Autodesk Inventor part; units mm, degrees
ref_plane "YZ Plane" through (0, 0, 0) normal (1, 0, 0) x (0, 1, 0)
ref_plane "XZ Plane" through (0, 0, 0) normal (0, 1, 0) x (-1, 0, 0)
ref_plane "XY Plane" through (0, 0, 0) normal (0, 0, 1) x (1, 0, 0)
sketch "Sketch1" plane through (0, 0, 0) normal (0, 0, 1) x (1, 0, 0)
  circle A0 centre (0, 0) radius 10
  arc A1 (13.8638, 0.9) -> (9.8638, 1.6449) centre (9.1431, -13.3378) ccw
  arc A2 (9.8638, -1.6449) -> (13.8638, -0.9) centre (9.1431, 13.3378) ccw
  arc A3 (13.8638, -0.9) -> (13.8638, 0.9) centre (-6.1159, 0) ccw
  line L0 (0, 0) -> (21.7354, 0) construction
  arc A4 (9.8638, -1.6449) -> (9.8638, 1.6449) centre (0, 0) ccw
  arc A5 (11.8575, 7.2397) -> (7.9696, 6.0404) centre (14.2942, -7.561) ccw
  arc A6 (12.694, 5.6459) -> (11.8575, 7.2397) centre (-5.4154, -2.8422) ccw
  arc A7 (9.4984, 3.1275) -> (12.694, 5.6459) centre (1.8975, 16.0591) ccw
  circle A8 centre (0, 0) radius 10
  arc A9 (9.4984, 3.1275) -> (7.9696, 6.0404) centre (0, 0) ccw
  arc A10 (7.1348, 11.9209) -> (4.2496, 9.0521) centre (16.1707, -0.0521) ccw
  arc A11 (8.6162, 10.8984) -> (7.1348, 11.9209) centre (-3.4743, -5.0333) ccw
  arc A12 (6.957, 7.1834) -> (8.6162, 10.8984) centre (-5.7829, 15.1014) ccw
  circle A13 centre (0, 0) radius 10
  arc A14 (6.957, 7.1834) -> (4.2496, 9.0521) centre (0, 0) ccw
  arc A15 (0.7777, 13.8712) -> (-0.4439, 9.9901) centre (14.3427, 7.4688) ccw
  arc A16 (2.5645, 13.6542) -> (0.7777, 13.8712) centre (-0.7372, -6.0714) ccw
  arc A17 (2.8218, 9.5936) -> (2.5645, 13.6542) centre (-12.1385, 10.6842) ccw
  circle A18 centre (0, 0) radius 10
  arc A19 (2.8218, 9.5936) -> (-0.4439, 9.9901) centre (0, 0) ccw
  arc A20 (-5.7577, 12.6437) -> (-5.0357, 8.6395) centre (9.2289, 13.2786) ccw
  arc A21 (-4.0747, 13.282) -> (-5.7577, 12.6437) centre (2.1687, -5.7185) ccw
  arc A22 (-1.9598, 9.8061) -> (-4.0747, 13.282) centre (-15.7133, 3.8193) ccw
  circle A23 centre (0, 0) radius 10
  arc A24 (-1.9598, 9.8061) -> (-5.0357, 8.6395) centre (0, 0) ccw
  arc A25 (-10.974, 8.5197) -> (-8.4739, 5.3097) centre (2.0009, 16.0465) ccw
  arc A26 (-9.7804, 9.8671) -> (-10.974, 8.5197) centre (4.5779, -4.0556) ccw
  arc A27 (-6.2924, 7.7721) -> (-9.7804, 9.8671) centre (-15.6884, -3.9205) ccw
  circle A28 centre (0, 0) radius 10
  arc A29 (-6.2924, 7.7721) -> (-8.4739, 5.3097) centre (0, 0) ccw
  arc A30 (-13.6763, 2.444) -> (-9.9708, 0.7635) centre (-5.6855, 15.1383) ccw
  arc A31 (-13.2456, 4.1917) -> (-13.6763, 2.444) centre (5.9382, -1.4636) ccw
  arc A32 (-9.1835, 3.9576) -> (-13.2456, 4.1917) centre (-12.0694, -10.7621) ccw
  circle A33 centre (0, 0) radius 10
  arc A34 (-9.1835, 3.9576) -> (-9.9708, 0.7635) centre (0, 0) ccw
  arc A35 (-13.2456, -4.1917) -> (-9.1835, -3.9576) centre (-12.0694, 10.7621) ccw
  arc A36 (-13.6763, -2.444) -> (-13.2456, -4.1917) centre (5.9382, 1.4636) ccw
  arc A37 (-9.9708, -0.7635) -> (-13.6763, -2.444) centre (-5.6855, -15.1383) ccw
  circle A38 centre (0, 0) radius 10
  arc A39 (-9.9708, -0.7635) -> (-9.1835, -3.9576) centre (0, 0) ccw
  arc A40 (-9.7804, -9.8671) -> (-6.2924, -7.7721) centre (-15.6884, 3.9205) ccw
  arc A41 (-10.974, -8.5197) -> (-9.7804, -9.8671) centre (4.5779, 4.0556) ccw
  arc A42 (-8.4739, -5.3097) -> (-10.974, -8.5197) centre (2.0009, -16.0465) ccw
  circle A43 centre (0, 0) radius 10
  arc A44 (-8.4739, -5.3097) -> (-6.2924, -7.7721) centre (0, 0) ccw
  arc A45 (-4.0747, -13.282) -> (-1.9598, -9.8061) centre (-15.7133, -3.8193) ccw
  arc A46 (-5.7577, -12.6437) -> (-4.0747, -13.282) centre (2.1687, 5.7185) ccw
  arc A47 (-5.0357, -8.6395) -> (-5.7577, -12.6437) centre (9.2289, -13.2786) ccw
  circle A48 centre (0, 0) radius 10
  arc A49 (-5.0357, -8.6395) -> (-1.9598, -9.8061) centre (0, 0) ccw
  arc A50 (2.5645, -13.6542) -> (2.8218, -9.5936) centre (-12.1385, -10.6842) ccw
  arc A51 (0.7777, -13.8712) -> (2.5645, -13.6542) centre (-0.7372, 6.0714) ccw
  arc A52 (-0.4439, -9.9901) -> (0.7777, -13.8712) centre (14.3427, -7.4688) ccw
  circle A53 centre (0, 0) radius 10
  arc A54 (-0.4439, -9.9901) -> (2.8218, -9.5936) centre (0, 0) ccw
  arc A55 (8.6162, -10.8984) -> (6.957, -7.1834) centre (-5.7829, -15.1014) ccw
  arc A56 (7.1348, -11.9209) -> (8.6162, -10.8984) centre (-3.4743, 5.0333) ccw
  arc A57 (4.2496, -9.0521) -> (7.1348, -11.9209) centre (16.1707, 0.0521) ccw
  circle A58 centre (0, 0) radius 10
  arc A59 (4.2496, -9.0521) -> (6.957, -7.1834) centre (0, 0) ccw
  arc A60 (12.694, -5.6459) -> (9.4984, -3.1275) centre (1.8975, -16.0591) ccw
  arc A61 (11.8575, -7.2397) -> (12.694, -5.6459) centre (-5.4154, 2.8422) ccw
  arc A62 (7.9696, -6.0404) -> (11.8575, -7.2397) centre (14.2942, 7.561) ccw
  circle A63 centre (0, 0) radius 10
  arc A64 (7.9696, -6.0404) -> (9.4984, -3.1275) centre (0, 0) ccw
  dimension "d0" = 20
  dimension "d3" = 15
  dimension "d4" = 15
  dimension "d5" = 4
  dimension "d6" = 20
  dimension "d7" = 1.8
  dimension "d10" = 360
extrude "Extrusion1" add sketch "Sketch1" along normal blind 10
sketch "Sketch2" plane through (0, 0, 10) normal (0, 0, 1) x (1, 0, 0)
  circle A0 centre (0, 0) radius 2.75
  dimension "d14" = 5.5
extrude "Extrusion2" cut sketch "Sketch2" against normal through all
sketch "Sketch3" plane through (0, 0, 0) normal (0, 0, -1) x (-1, 0, 0)
  circle A0 centre (0, 0) radius 17.5
  circle A1 centre (0, 0) radius 3.2083
  dimension "d17" = 35
extrude "Extrusion3" add sketch "Sketch3" along normal blind 5
properties part number "BA006" material "ABS Plastic"
Geometry: final body of the model. Coordinates: model frame, mm. A direction names the side the tool comes from. Round coordinates to 2 decimals unless told otherwise and drop trailing zeros. Order: outer loops, then holes, each group sorted by start corner. A loop starts at its lowest first (then second) coordinate and runs counter-clockwise, first axis right, second up. Notation, with made-up numbers: (23.25, 88.5) -> (52.25, 88.5) arc R18 cw to (52.25, 109.5) -> close; hole circle Ø1 at (66.25, 28.5). An arc over 180 degrees is marked (long way). Use CSV: the item, a comma, the result in double quotes. Start each with the question number.
1) Draft query along Y for faces 1 (the face through (7.492, -6.623, 4.93)), 2 (the face through (-0.596, -2.685, 5.07)), 3 (the face through (-10.4, 9.2, 4.9)), 4 (the face through (-13.48, -3.33, 4.93)). Return one class per face: +Y half, -Y half, draft (parallel to the pull), parting line (faces both ways), or undercut.
2) Set-up query: faces 5 (the face through (-6, 8, 5)), 6 (the face through (-2.884, -11.592, 4.93)), 7 (the face through (12.29, 6.46, 4.93)). Return all of +Z, -Z, +X, -X, +Y, -Y with unobstructed straight access to the full face (end or side cutting, diameter ignored); none if empty.
3) First-contact query: pin 1 Ø1 at (y, z) = (5.5, 0) entering from +X; pin 2 Ø4 at (y, z) = (10.5, -2) entering from +X; pin 3 Ø7.5 at (x, y) = (0, 0) entering from -Z; pin 4 Ø2 at (x, z) = (2.5, 4.5) entering from +Y. Flat tips, straight axial feed; report the tip coordinate or a pass-through.
4) Section C-C (y = -6.5). Return the cut outline in (x, z).
5) Material intervals for line 1 along X through (y, z) = (-10.5, 7.75); line 2 along Y through (x, z) = (0, -3.9); line 3 along Y through (x, z) = (8, 2.5), sorted ascending. Write a range as from..to.
6) Section D-D (x = -4.5). Return the cut outline in (y, z), and give its area (3 significant figures).
7) Section B-B (x = 0). Return the cut outline in (y, z).
8) Section A-A (y = 0). Return the cut outline in (x, z).
Returned:
1,face 1,"undercut"
1,face 2,"undercut"
1,face 3,"+Y half"
1,face 4,"-Y half"
2,face 5,"+Z"
2,face 6,"+Z, -Y"
2,face 7,"+Z, +X, +Y"
3,pin 1,"stops at x = 16.77"
3,pin 2,"stops at x = 15.3"
3,pin 3,"stops at z = -5"
3,pin 4,"stops at y = 13.8"
4,outline,"(-16.25, -5) -> (16.25, -5) -> (16.25, 0) -> (12.27, 0) -> (12.27, 10) -> (9.07, 10) -> (9.07, 0) -> (7.6, 0) -> (7.6, 10) -> (-9.57, 10) -> (-9.57, 0) -> (-16.25, 0) -> close"
5,line 1,"x = -5.51..-2.28, -0.35..2.86, 5.51..8.49"
5,line 2,"y = -17.5..-3.21, 3.21..17.5"
5,line 3,"y = -11.35..-9.18, -6.05..6.05, 9.18..11.35"
6,outline,"(-16.91, -5) -> (16.91, -5) -> (16.91, 0) -> (13.14, 0) -> (13.14, 10) -> (-13.14, 10) -> (-13.14, 0) -> (-16.91, 0) -> close"
6,area,"432 mm²"
7,outline,"(-17.5, -5) -> (-3.21, -5) -> (-3.21, 0) -> (-2.75, 0) -> (-2.75, 10) -> (-11.86, 10) -> (-11.86, 0) -> (-17.5, 0) -> close; (2.75, 0) -> (3.21, 0) -> (3.21, -5) -> (17.5, -5) -> (17.5, 0) -> (11.86, 0) -> (11.86, 10) -> (2.75, 10) -> close"
8,outline,"(-17.5, -5) -> (-3.21, -5) -> (-3.21, 0) -> (-2.75, 0) -> (-2.75, 10) -> (-10, 10) -> (-10, 0) -> (-17.5, 0) -> close; (2.75, 0) -> (3.21, 0) -> (3.21, -5) -> (17.5, -5) -> (17.5, 0) -> (13.88, 0) -> (13.88, 10) -> (2.75, 10) -> close"
